from build123d import *

# Parameters (mm, degrees)
BOSS_EXTRUDE1_DEPTH      = 2.5
SKETCH24_R               = 1.534588162
SKETCH24_R_2             = 1.539679215
SKETCH24_R_3             = 1.53510928
SKETCH24_R_4             = 1.507254119
SKETCH24_R_5             = 1.501766116
SKETCH24_R_6             = 1.506723366
CUT_EXTRUDE7_DEPTH       = 1
CUT_EXTRUDE7_DEPTH_BACK  = 3.5
SKETCH28_R               = 4.5
SKETCH28_R_2             = 1.5
BOSS_EXTRUDE4_DEPTH      = 5
SKETCH29_R               = 1.5
CUT_EXTRUDE10_DEPTH      = 6
CUT_EXTRUDE10_DEPTH_BACK = 3.5
SKETCH30_W               = 39
SKETCH30_H               = 18
BOSS_EXTRUDE5_DEPTH      = 30
CUT_EXTRUDE11_DEPTH      = 32.629888849
SKETCH32_R               = 3.11925
SKETCH32_R_2             = 1.61925
SKETCH32_R_3             = 3.25
SKETCH32_R_4             = 1.75
SKETCH32_R_5             = 3.255054338
SKETCH32_R_6             = 1.755054338
BOSS_EXTRUDE6_DEPTH      = 3.5
SKETCH33_R               = 1.755054338
SKETCH33_R_2             = 1.75
SKETCH33_R_3             = 1.61925
CUT_EXTRUDE12_DEPTH      = 31
CUT_EXTRUDE12_DEPTH_BACK = 3.5
SKETCH34_W               = 35.425074467
SKETCH34_H               = 46.294311582
SKETCH34_W_2             = 13.394736858
SKETCH34_H_2             = 25.79034775
SKETCH34_W_3             = 19.34309219
SKETCH34_H_3             = 32.937244524
SKETCH34_W_4             = 12.732315529
SKETCH34_H_4             = 15
SKETCH34_W_5             = 11.855681534
CUT_EXTRUDE13_DEPTH      = 3.5
SKETCH35_W               = 1.308538477
SKETCH35_H               = 100
BOSS_EXTRUDE7_DEPTH      = 2.5


with BuildPart() as part:
    # Sketch2 → Boss-Extrude1 (new body)
    with BuildSketch(Plane(origin=(0, -17.332299444, 0), x_dir=(-1, 0, 0), z_dir=(0, -1, 0))):
        Polygon((-29.674557938, 41.468970044), (-48.61030302, 16.085172631), (-48.61030302, -34.61356185), (-29.352965282, -58.531029956), (-29.352965282, -66.036105098), (-19.352967368, -66.036105098), (-19.352967368, -58.531029956), (43.147035426, -58.531029956), (43.147035426, -66.036105098), (53.147035202, -66.036105098), (53.147035202, -58.531029956), (115.647037996, -58.531029956), (115.647037996, -66.036105098), (125.241603418, -66.036105098), (125.241603418, -58.531029956), (145.143417646, -58.531029956), (145.143417646, 41.468970044), (125.241603418, 41.468970044), (125.241603418, 48.975336237), (115.668802349, 48.975336237), (115.668802349, 41.468970044), (53.135946408, 41.468970044), (53.135946408, 48.975336237), (43.168799778, 48.975336237), (43.168799778, 41.468970044), (-19.254443916, 41.468970044), (-19.254443916, 48.975336237), (-29.674557938, 48.975336237), align=None)
    extrude(amount=-BOSS_EXTRUDE1_DEPTH)

    # Sketch24 → Cut-Extrude7 (cut, two sides)
    with BuildSketch(Plane(origin=(0, -14.832299444, 0), x_dir=(1, 0, 0), z_dir=(0, 1, 0))) as cut_extrude7_sk:
        with Locations((-120.631514326, 43.936289371)):
            Circle(SKETCH24_R)
        with Locations((-48.193182725, 43.936289371)):
            Circle(SKETCH24_R_2)
        with Locations((24.374871647, 43.936289371)):
            Circle(SKETCH24_R_3)
        with Locations((24.374871647, -61.035755979)):
            Circle(SKETCH24_R_4)
        with Locations((-48.193182725, -61.035755979)):
            Circle(SKETCH24_R_5)
        with Locations((-120.631514326, -61.035755979)):
            Circle(SKETCH24_R_6)
    extrude(amount=CUT_EXTRUDE7_DEPTH, mode=Mode.SUBTRACT)
    extrude(cut_extrude7_sk.sketch, amount=-CUT_EXTRUDE7_DEPTH_BACK, mode=Mode.SUBTRACT)

    # Sketch28 → Boss-Extrude4 (add)
    with BuildSketch(Plane(origin=(0, -14.832299444, 0), x_dir=(1, 0, 0), z_dir=(0, 1, 0))):
        with Locations((44.095100387, -18.794047136)):
            Circle(SKETCH28_R)
        with Locations((44.095100387, -18.794047136)):
            Circle(SKETCH28_R_2, mode=Mode.SUBTRACT)
        with Locations((44.095100387, 2.033952864)):
            Circle(SKETCH28_R)
        with Locations((44.095100387, 2.033952864)):
            Circle(SKETCH28_R_2, mode=Mode.SUBTRACT)
        with Locations((31.687794159, 2.033952864)):
            Circle(SKETCH28_R)
        with Locations((31.687794159, 2.033952864)):
            Circle(SKETCH28_R_2, mode=Mode.SUBTRACT)
        with Locations((31.687794159, -18.794047136)):
            Circle(SKETCH28_R)
        with Locations((31.687794159, -18.794047136)):
            Circle(SKETCH28_R_2, mode=Mode.SUBTRACT)
        with Locations((20.460418505, 2.033952864)):
            Circle(SKETCH28_R)
        with Locations((20.460418505, 2.033952864)):
            Circle(SKETCH28_R_2, mode=Mode.SUBTRACT)
        with Locations((20.460418505, -18.794047136)):
            Circle(SKETCH28_R)
        with Locations((20.460418505, -18.794047136)):
            Circle(SKETCH28_R_2, mode=Mode.SUBTRACT)
    extrude(amount=BOSS_EXTRUDE4_DEPTH)

    # Sketch29 → Cut-Extrude10 (cut, two sides)
    with BuildSketch(Plane(origin=(0, -14.832299444, 0), x_dir=(1, 0, 0), z_dir=(0, 1, 0))) as cut_extrude10_sk:
        with Locations((44.095100387, -18.794047136)):
            Circle(SKETCH29_R)
        with Locations((44.095100387, 2.033952864)):
            Circle(SKETCH29_R)
        with Locations((20.460418505, -18.794047136)):
            Circle(SKETCH29_R)
        with Locations((20.460418505, 2.033952864)):
            Circle(SKETCH29_R)
        with Locations((31.687794159, 2.033952864)):
            Circle(SKETCH29_R)
        with Locations((31.687794159, -18.794047136)):
            Circle(SKETCH29_R)
    extrude(amount=CUT_EXTRUDE10_DEPTH, mode=Mode.SUBTRACT)
    extrude(cut_extrude10_sk.sketch, amount=-CUT_EXTRUDE10_DEPTH_BACK, mode=Mode.SUBTRACT)

    # Sketch30 → Boss-Extrude5 (add)
    with BuildSketch(Plane(origin=(0, -14.832299444, 0), x_dir=(1, 0, 0), z_dir=(0, 1, 0))):
        with Locations((-5.862319178, -43.406216249)):
            Rectangle(SKETCH30_W, SKETCH30_H)
    extrude(amount=BOSS_EXTRUDE5_DEPTH)

    # Sketch31 → Cut-Extrude11 (cut, through all)
    with BuildSketch(Plane(origin=(0, 0, 34.406216249), x_dir=(-1, 0, 0), z_dir=(0, 0, -1))):
        Polygon((-10.637680822, -11.832299444), (-10.637680822, -14.832299444), (22.362319178, -14.832299444), (22.362319178, -11.832299444), (22.362319178, 12.167700556), (-10.637680822, 12.167700556), align=None)
    extrude(amount=-CUT_EXTRUDE11_DEPTH, mode=Mode.SUBTRACT)

    # Sketch32 → Boss-Extrude6 (add)
    with BuildSketch(Plane(origin=(0, -14.832299444, 0), x_dir=(1, 0, 0), z_dir=(0, 1, 0))):
        with Locations((-78.332170896, -22.386024774)):
            Circle(SKETCH32_R)
        with Locations((-78.332170896, -22.386024774)):
            Circle(SKETCH32_R_2, mode=Mode.SUBTRACT)
        with Locations((-63.092170896, 28.401275226)):
            Circle(SKETCH32_R)
        with Locations((-63.092170896, 28.401275226)):
            Circle(SKETCH32_R_2, mode=Mode.SUBTRACT)
        with Locations((-35.164870896, 28.401275226)):
            Circle(SKETCH32_R)
        with Locations((-35.164870896, 28.401275226)):
            Circle(SKETCH32_R_2, mode=Mode.SUBTRACT)
        with Locations((-30.415070896, -23.529024774)):
            Circle(SKETCH32_R)
        with Locations((-30.415070896, -23.529024774)):
            Circle(SKETCH32_R_2, mode=Mode.SUBTRACT)
        with Locations((5.365042011, 25.69595377)):
            Circle(SKETCH32_R_3)
        with Locations((5.365042011, 25.69595377)):
            Circle(SKETCH32_R_4, mode=Mode.SUBTRACT)
        with Locations((5.365042011, -9.30404623)):
            Circle(SKETCH32_R_3)
        with Locations((5.365042011, -9.30404623)):
            Circle(SKETCH32_R_4, mode=Mode.SUBTRACT)
        with Locations((-17.634957989, -9.30404623)):
            Circle(SKETCH32_R_5)
        with Locations((-17.634957989, -9.30404623)):
            Circle(SKETCH32_R_6, mode=Mode.SUBTRACT)
        with Locations((-17.634957989, 25.69595377)):
            Circle(SKETCH32_R_5)
        with Locations((-17.634957989, 25.69595377)):
            Circle(SKETCH32_R_6, mode=Mode.SUBTRACT)
    extrude(amount=BOSS_EXTRUDE6_DEPTH)

    # Sketch33 → Cut-Extrude12 (cut, two sides)
    with BuildSketch(Plane(origin=(0, -14.832299444, 0), x_dir=(1, 0, 0), z_dir=(0, 1, 0))) as cut_extrude12_sk:
        with Locations((-17.634957989, 25.69595377)):
            Circle(SKETCH33_R)
        with Locations((-17.634957989, -9.30404623)):
            Circle(SKETCH33_R)
        with Locations((5.365042011, -9.30404623)):
            Circle(SKETCH33_R_2)
        with Locations((5.365042011, 25.69595377)):
            Circle(SKETCH33_R_2)
        with Locations((-78.332170896, -22.386024774)):
            Circle(SKETCH33_R_3)
        with Locations((-63.092170896, 28.401275226)):
            Circle(SKETCH33_R_3)
        with Locations((-35.164870896, 28.401275226)):
            Circle(SKETCH33_R_3)
        with Locations((-30.415070896, -23.529024774)):
            Circle(SKETCH33_R_3)
    extrude(amount=CUT_EXTRUDE12_DEPTH, mode=Mode.SUBTRACT)
    extrude(cut_extrude12_sk.sketch, amount=-CUT_EXTRUDE12_DEPTH_BACK, mode=Mode.SUBTRACT)

    # Sketch34 → Cut-Extrude13 (cut, through all)
    with BuildSketch(Plane(origin=(0, -14.832299444, 0), x_dir=(1, 0, 0), z_dir=(0, 1, 0))):
        with Locations((-55.089850794, -1.917647795)):
            Rectangle(SKETCH34_W, SKETCH34_H)
        with Locations((-6.697368429, 8.334334121)):
            Rectangle(SKETCH34_W_2, SKETCH34_H_2)
        with Locations((-5.977817897, -33.923153054)):
            Rectangle(SKETCH34_W_3, SKETCH34_H_3)
        with Locations((27.139734393, 22.033952864)):
            Rectangle(SKETCH34_W_4, SKETCH34_H_4)
        with Locations((26.701417396, -38.794047136)):
            Rectangle(SKETCH34_W_5, SKETCH34_H_4)
    extrude(amount=-CUT_EXTRUDE13_DEPTH, mode=Mode.SUBTRACT)

    # Sketch35 → Boss-Extrude7 (add)
    with BuildSketch(Plane(origin=(0, -14.832299444, 0), x_dir=(1, 0, 0), z_dir=(0, 1, 0))):
        with Locations((-144.489148408, -8.531029956)):
            Rectangle(SKETCH35_W, SKETCH35_H)
    extrude(amount=BOSS_EXTRUDE7_DEPTH)


solid = part.part
Work out the finished part from the listing and answer in its coordinate system (mm). A direction names the side the tool comes from. Give positions to 0.01 mm unless a question says otherwise; leave off trailing zeros. Write each loop counter-clockwise with the first axis right and the second up, starting at its lowest first coordinate (ties: lowest second). Pieces come first, ordered by that corner, then holes. Notation, with made-up numbers: (63.5, -13) - (111.5, -13) arc R20 cw to (111.5, 11) - close; hole circle Ø7 at (41.25, 78.25). An arc over 180 degrees is marked (long way). One line per item, written item: value. Start each with the question number.
1. Consider probe 1 along X at (y, z) = (-14, 45.5); probe 2 along Y at (x, z) = (-99, 48.5); probe 3 along X at (y, z) = (-14.5, 13). Determine where each line is inside the solid, lowest interval first.
2. Find section C-C (z = -37.5). Write down the section's boundary in (x, y), then the cut area to 3 significant figures.
3. Find section A-A (y = -4). Write down the section's boundary in (x, z).
4. For faces 1 (the cylindrical face through (-38.28, -13.11, -28.54)), 2 (the flat face through (-29, -11.332, 25)), 3 (the flat face through (10.638, -1, 43)), 4 (the flat face through (-135, -16, 58.531)), determine the directions among +Z, -Z, +X, -X, +Y, -Y from which every point of the face is accessible in a straight line to the end or side of a thin tool.
5. Find section B-B (z = 37). Write down the section's boundary in (x, y).
6. Given pin 1 (8 mm diameter, centred on y = -3.5, z = 43, fed in from +X); pin 2 (5 mm diameter, centred on x = -36, z = -28, fed in from +Y); pin 3 (9 mm diameter, centred on y = -3.5, z = 44, fed in from -X); pin 4 (2 mm diameter, centred on x = -17.63, z = -25.7, fed in from +Y), each flat-ended and moving along its own axis, determine where each tip first touches the part or whether it passes through.
7. For a pull along X with two mould halves and no side action, classify faces 5 (the cylindrical face through (48.387, -12.367, -3.386)), 6 (the flat face through (-4.51, 12.32, 34.406)) as +X half, -X half, draft (parallel to the pull), parting line (faces both ways), or undercut.
Geometry results:
1. probe 1: -145.14 to -143.83, -25.36 to -22.36, 10.64 to 13.64
1. probe 2: -17.33 to -14.83
1. probe 3: -145.14 to -143.83
2. outline: (-145.14, -17.33) - (32.64, -17.33) - (32.64, -14.83) - (-143.83, -14.83) - (-143.83, -12.33) - (-145.14, -12.33) - close
2. area: 448 mm2
3. outline: (-25.36, 34.41) - (-22.36, 34.41) - (-22.36, 52.41) - (-25.36, 52.41) - close; (10.64, 34.41) - (13.64, 34.41) - (13.64, 52.41) - (10.64, 52.41) - close
4. face 1: +Y
4. face 2: +Z, -Z, -X, +Y
4. face 3: +Z, -Z
4. face 4: +Z, -X, +Y, -Y
5. outline: (-145.14, -17.33) - (-15.65, -17.33) - (-15.65, -14.83) - (-22.36, -14.83) - (-22.36, 12.17) - (10.64, 12.17) - (10.64, -14.83) - (3.69, -14.83) - (3.69, -17.33) - (20.77, -17.33) - (20.77, -14.83) - (13.64, -14.83) - (13.64, 15.17) - (-25.36, 15.17) - (-25.36, -14.83) - (-143.83, -14.83) - (-143.83, -12.33) - (-145.14, -12.33) - close; (32.63, -17.33) - (46.69, -17.33) - (46.69, -14.83) - (32.63, -14.83) - close
6. pin 1: x = 13.64
6. pin 2: y = -11.33
6. pin 3: x = -25.36
6. pin 4: through
7. face 5: undercut
7. face 6: draft
